Study the drawing (mm; zero at the part's minimum x, y, z) and answer. A direction names the side the tool comes from. Coordinates: 2 decimals unless noted, no trailing zeros. Order: outer loops, then holes, each group sorted by start corner. A loop starts at its lowest first (then second) coordinate and runs counter-clockwise, first axis right, second up. Notation, with made-up numbers: (53, -28) -> (103, -28) arc R19 ccw to (103, -24) -> close; hole circle Ø3 at (-23.75, 7). An arc over 180 degrees is marked (long way). Write each question's results on one line, items separated by ' | '. Start each with the question number.
(1) The part is cut by section C-C, the plane z = 14.75. Give the vertices of the cut face in (x, y).
(2) Determine the mould class of the marked faces 1, 2, 3 and 4 for opening direction Z: +Z half, -Z half, draft (parallel to the pull), parting line (faces both ways), or undercut.
(3) Straight lines are drawn through the part: L1, parallel to Y at x = 8, z = 5.5; L2, parallel to Z at x = 14.75, y = 8; L3, parallel to Y at x = 8, z = 9. For each, find the intervals that lie inside material, in ascending order.
(4) The part is cut by section D-D, the plane x = 4.75. Give the vertices of the cut face in (y, z), then the cut area to 3 significant figures.
(5) The part is cut by section A-A, the plane x = 8. Give the vertices of the cut face in (y, z).
(6) Given pin 1 (8 mm diameter, centred on x = 6.5, y = 7, fed in from +Z); pin 2 (3 mm diameter, centred on x = 5, z = 12, fed in from +Y); pin 3 (4 mm diameter, centred on x = 2, z = 9, fed in from +Y); pin 4 (5 mm diameter, centred on y = 12, z = 9.5, fed in from +X), each flat-ended and moving along its own axis, determine where each tip first touches the part or whether it passes through.
(7) A tool of negligible diameter and unlimited length cuts with its end or side. For the marked faces 5 and 6, from which of +Z, -Z, +X, -X, +Y, -Y can it reach the whole face along a straight path? Write none if from no direction.
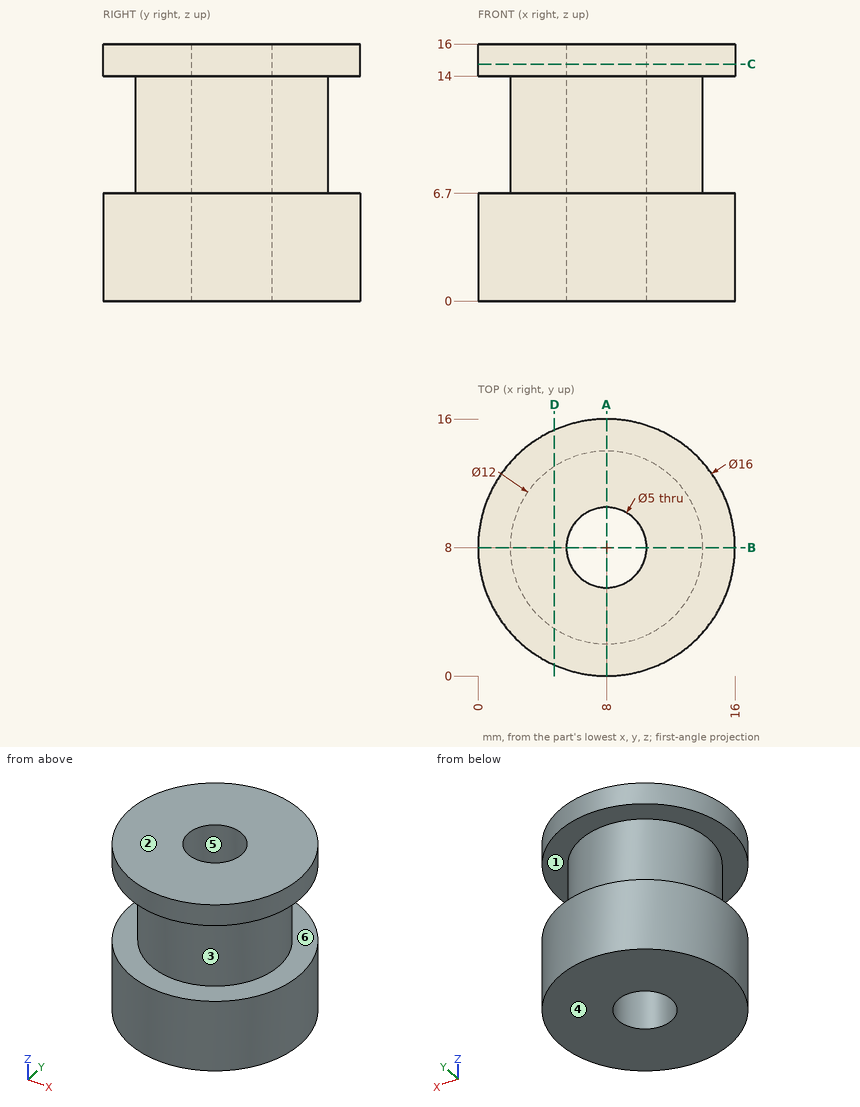
Established:
1) outline: circle Ø16 at (8, 8); hole circle Ø5 at (8, 8)
2) face 1: undercut | face 2: +Z half | face 3: undercut | face 4: -Z half
3) L1: y = 0 to 5.5, 10.5 to 16 | L2: z = 0 to 6.7, 14 to 16 | L3: y = 2 to 5.5, 10.5 to 14
4) outline: (0.69, 0) -> (15.31, 0) -> (15.31, 6.7) -> (13.04, 6.7) -> (13.04, 14) -> (15.31, 14) -> (15.31, 16) -> (0.69, 16) -> (0.69, 14) -> (2.96, 14) -> (2.96, 6.7) -> (0.69, 6.7) -> close | area: 201 mm^2
5) outline: (0, 0) -> (5.5, 0) -> (5.5, 16) -> (0, 16) -> (0, 14) -> (2, 14) -> (2, 6.7) -> (0, 6.7) -> close; (10.5, 0) -> (16, 0) -> (16, 6.7) -> (14, 6.7) -> (14, 14) -> (16, 14) -> (16, 16) -> (10.5, 16) -> close
6) pin 1: stops at z = 16 | pin 2: stops at y = 13.81 | pin 3: stops at y = 12.47 | pin 4: stops at x = 13.81
7) face 5: +Z, -Z | face 6: none
